```python
from build123d import *

# Parameters (mm, degrees)
F0_R     = 6.000001
F1_DEPTH = 38.999922
F2_R     = 2.149996
F3_DEPTH = 39.751
F4_R     = 11.000003
F4_R_2   = 6.000001
F5_DEPTH = 2.999994
F6_R     = 10.9982
F6_R_2   = 6.000001
F7_DEPTH = 2.999994


with BuildPart() as f1:
    # F0 (on Front) → F1 (new body)
    with BuildSketch(Plane.XZ):
        Polygon((-23.076807, 21.293776), (-25.046914, 19.794005), (-25.046914, 13.42603), (-23.546917, 11.456095), (-23.546917, -9.2142), (-13.846911, -9.2142), (-10.296957, -13.185778), (2.203044, -13.185778), (5.752999, -9.2142), (15.453005, -9.2142), (15.453005, 11.456095), (16.953002, 13.42603), (16.953002, 19.794005), (14.949928, 21.249454), (7.756072, 21.249454), (5.752999, 19.794005), (-13.846911, 19.794005), (-15.849985, 21.249454), align=None)
        with Locations((-4.128998, 6.249459)):
            Circle(F0_R, mode=Mode.SUBTRACT)
    extrude(amount=F1_DEPTH)

    # F2 (on face) → F3 (cut, symmetric)
    with BuildSketch(Plane.XY.offset(19.794005)):
        with Locations((-19.276814, -6.892563)):
            Circle(F2_R)
        with Locations((-19.276814, -32.107359)):
            Circle(F2_R)
        with Locations((11.182902, -6.892563)):
            Circle(F2_R)
        with Locations((11.182902, -32.107359)):
            Circle(F2_R)
    extrude(amount=F3_DEPTH, both=True, mode=Mode.SUBTRACT)

    # F4 (on face) → F5 (cut)
    with BuildSketch(Plane(origin=(0, 0, 0), x_dir=(-1, 0, 0), z_dir=(0, 1, 0))):
        with Locations((4.128998, 6.249459)):
            Circle(F4_R)
        with Locations((4.128998, 6.249459)):
            Circle(F4_R_2, mode=Mode.SUBTRACT)
    extrude(amount=-F5_DEPTH, mode=Mode.SUBTRACT)

    # F6 (on face) → F7 (cut)
    with BuildSketch(Plane.XZ.offset(38.999922)):
        with Locations((-4.128998, 6.249459)):
            Circle(F6_R)
        with Locations((-4.128998, 6.249459)):
            Circle(F6_R_2, mode=Mode.SUBTRACT)
    extrude(amount=-F7_DEPTH, mode=Mode.SUBTRACT)


solid = f1.part
```
Design review of the part built by this model. Coordinates are the model's own, in mm. A direction names the side the tool comes from. Give positions to 0.01 mm unless a question says otherwise; leave off trailing zeros. Order: outer loops, then holes, each group sorted by start corner. A loop starts at its lowest first (then second) coordinate and runs counter-clockwise, first axis right, second up. Notation, with made-up numbers: (84, 37.5) - (99, 37.5) arc R28 ccw to (99, 68.5) - close; hole circle Ø5 at (-15.75, 13.25). An arc over 180 degrees is marked (long way). Use a Markdown table: item, result. Add a question column.
(1) Add section D-D on z = -7. Give the boundary of the cut face in (x, y).
(2) Mouldability with a two-part tool opening along Z and no side actions: class faces 6 (the face through (-6.513, -37.521, -4.487)), 7 (the face through (10.903, -29.976, 6.231)), 8 (the face through (-24.307, -19.227, 12.455)) as +Z half, -Z half, draft (parallel to the pull), parting line (faces both ways), or undercut.
(3) Wall thickness on probe 1 along Y at (x, z) = (-18.5, -2); probe 2 along X at (y, z) = (-18.5, 0); probe 3 along Z at (x, y) = (14.5, -22): over which ranges is each line inside the solid? List them lowest first. Write a range as [from, to].
(4) Clearance check with flat-ended pins moving along their axes: P1, Ø2, axis at x = -11.5, z = 2.5, coming from the -Y side; P2, Ø4, axis at x = -6.5, y = -27.5, coming from the +Z side; P3, Ø5.5, axis at x = 11.18, y = -6.89, coming from the -Z side. State where each tip first meets the part, or that it passes through.
(5) Add section C-C on x = -5. Give the boundary of the cut face in (y, z), then the cut area to 3 significant figures.
(6) Add section A-A on y = -31. Give the boundary of the cut face in (x, z).
(7) Add section B-B on z = 8.5. Give the boundary of the cut face in (x, y), then the cut area to 3 significant figures.
(8) Machinability: for faces 1 (the face through (-23.547, -19, 1)), 2 (the face through (-25.047, -19, 17)), 3 (the face through (6.769, -19.227, 20.532)), 4 (the face through (15.453, -19, 1)), 5 (the face through (-4, -19, -13.186)), which of the approach directions +Z, -Z, +X, -X, +Y, -Y give a long, thin tool a straight path to every point of the face, cutting with its end or side? Answer none if there is none.
Report:
| question | item | result |
|---|---|---|
| 1 | outline | (-23.55, -39) - (15.45, -39) - (15.45, 0) - (-23.55, 0) - close; hole circle Ø4.3 at (-19.28, -32.11); hole circle Ø4.3 at (-19.28, -6.89); hole circle Ø4.3 at (11.18, -32.11); hole circle Ø4.3 at (11.18, -6.89) |
| 2 | face 6 | undercut |
| 2 | face 7 | draft |
| 2 | face 8 | -Z half |
| 3 | probe 1 | y = [-39, -34.11], [-30.1, -8.9], [-4.89, 0] |
| 3 | probe 2 | x = [-23.55, 15.45] |
| 3 | probe 3 | z = [-9.21, 21.25] |
| 4 | P1 | stops at y = -36 |
| 4 | P2 | stops at z = 19.79 |
| 4 | P3 | stops at z = -9.21 |
| 5 | outline | (-39, -13.19) - (0, -13.19) - (0, -4.72) - (-3, -4.72) - (-3, 0.31) - (-36, 0.31) - (-36, -4.71) - (-39, -4.71) - close; (-39, 17.21) - (-36, 17.21) - (-36, 12.19) - (-3, 12.19) - (-3, 17.21) - (0, 17.21) - (0, 19.79) - (-39, 19.79) - close |
| 5 | area | 763 mm² |
| 6 | outline | (-25.05, 13.43) - (-23.55, 11.46) - (-23.55, -9.21) - (-21.12, -9.21) - (-21.12, 21.28) - (-23.08, 21.29) - (-25.05, 19.79) - close; (-17.43, -9.21) - (-13.85, -9.21) - (-10.3, -13.19) - (2.2, -13.19) - (5.75, -9.21) - (9.34, -9.21) - (9.34, 21.25) - (7.76, 21.25) - (5.75, 19.79) - (-13.85, 19.79) - (-15.85, 21.25) - (-17.43, 21.26) - close; (13.03, -9.21) - (15.45, -9.21) - (15.45, 11.46) - (16.95, 13.43) - (16.95, 19.79) - (14.95, 21.25) - (13.03, 21.25) - close; hole circle Ø12 at (-4.13, 6.25) |
| 7 | outline | (-23.55, -39) - (-14.89, -39) - (-14.89, -36) - (-9.69, -36) - (-9.69, -3) - (-14.9, -3) - (-14.9, 0) - (-23.55, 0) - close; (1.43, -36) - (6.64, -36) - (6.64, -39) - (15.45, -39) - (15.45, 0) - (6.64, 0) - (6.64, -3) - (1.43, -3) - close; hole circle Ø4.3 at (-19.28, -32.11); hole circle Ø4.3 at (-19.28, -6.89); hole circle Ø4.3 at (11.18, -32.11); hole circle Ø4.3 at (11.18, -6.89) |
| 7 | area | 967 mm² |
| 8 | face 1 | -Z, -X, +Y, -Y |
| 8 | face 2 | +Z, -Z, -X, +Y, -Y |
| 8 | face 3 | +Z, +Y, -Y |
| 8 | face 4 | -Z, +X, +Y, -Y |
| 8 | face 5 | -Z, +X, -X, +Y, -Y |
